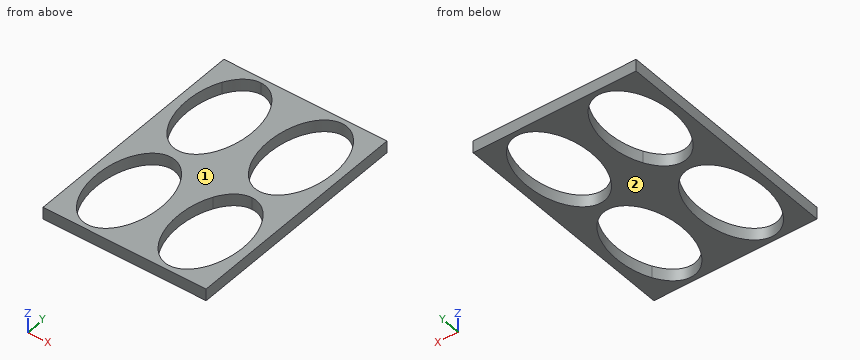
Autodesk Inventor part; units mm, degrees
ref_plane "YZ Plane" through (0, 0, 0) normal (1, 0, 0) x (0, 1, 0)
ref_plane "XZ Plane" through (0, 0, 0) normal (0, 1, 0) x (-1, 0, 0)
ref_plane "XY Plane" through (0, 0, 0) normal (0, 0, 1) x (1, 0, 0)
sketch "Эскиз1" plane through (0, 0, 0) normal (0, 0, 1) x (1, 0, 0)
  line L0 (0, 0) -> (218, 0)
  line L1 (218, 0) -> (218, -309)
  line L2 (218, -309) -> (0, -309)
  line L3 (0, -309) -> (0, 0)
  line L4 (0, 0) -> (218, -309)
  line L5 (218, 0) -> (0, -309) construction
  line L6 (0, -154.5) -> (218, -154.5) construction
  line L7 (109, 0) -> (109, -309) construction
  line L8 (109, 0) -> (0, -154.5) construction
  line L9 (0, -154.5) -> (109, -309) construction
  line L10 (109, -309) -> (218, -154.5) construction
  line L11 (218, -154.5) -> (109, 0) construction
  ellipse E0 centre (163.5, -231.75) end of major axis (163.5, -161.0034) minor radius 43.2868
  ellipse E1 centre (54.5, -231.75) end of major axis (54.5, -161.0034) minor radius 43.2868
  ellipse E2 centre (163.5, -77.25) end of major axis (163.5, -6.5034) minor radius 43.2868
  ellipse E3 centre (54.5, -77.25) end of major axis (54.5, -6.5034) minor radius 43.2868
  dimension "d0" = 218
  dimension "d1" = 309
extrude "Выдавливание2" add sketch "Эскиз1" along normal blind 16 contours L4 E3 E0 L2 L3 | L0 L1 L4 E0 E3
properties part number "ArmDesk" material "Древесно-стружечная плита"
Read the model definition and answer for the solid it produces. Units are mm, in the model's axes. Face numbers are marked on the shaded views. Coordinates: 2 decimals unless noted, no trailing zeros. Return JSON: item names as keys, results as strings.
(1) For a pull along Z with two mould halves and no side action, classify the marked faces 1 and 2 as pulls with the +Z half, pulls with the -Z half, needs draft (parallel to the pull), parting line crosses it, or undercut.
Answers below:
{"face 1": "pulls with the +Z half", "face 2": "pulls with the -Z half"}
(2) Consider line 1 along X through (y, z) = (-229, 6.75); line 2 along Y through (x, z) = (20.5, 6). Determine where each line is inside the solid, lowest interval first. Write a range as from..to.
Answers below:
{"line 1": "0..11.25, 97.75..120.25, 206.75..218", "line 2": "-309..-275.54, -187.96..-121.04, -33.46..0"}
(3) The part is cut by section A-A on z = 7. State how many separate pieces and enclosed holes the cut face has, then the cut area to 3 significant figures.
Answers below:
{"separate pieces": "1", "enclosed holes": "4", "area": "28,900 mm^2"}
